Geometry check sheet. Reference: drawing and pictorial views, mm from the part's lowest x, y, z. A direction names the side the tool comes from. Give positions to 0.01 mm unless a question says otherwise; leave off trailing zeros. Write each loop counter-clockwise with the first axis right and the second up, starting at its lowest first coordinate (ties: lowest second). Pieces come first, ordered by that corner, then holes.
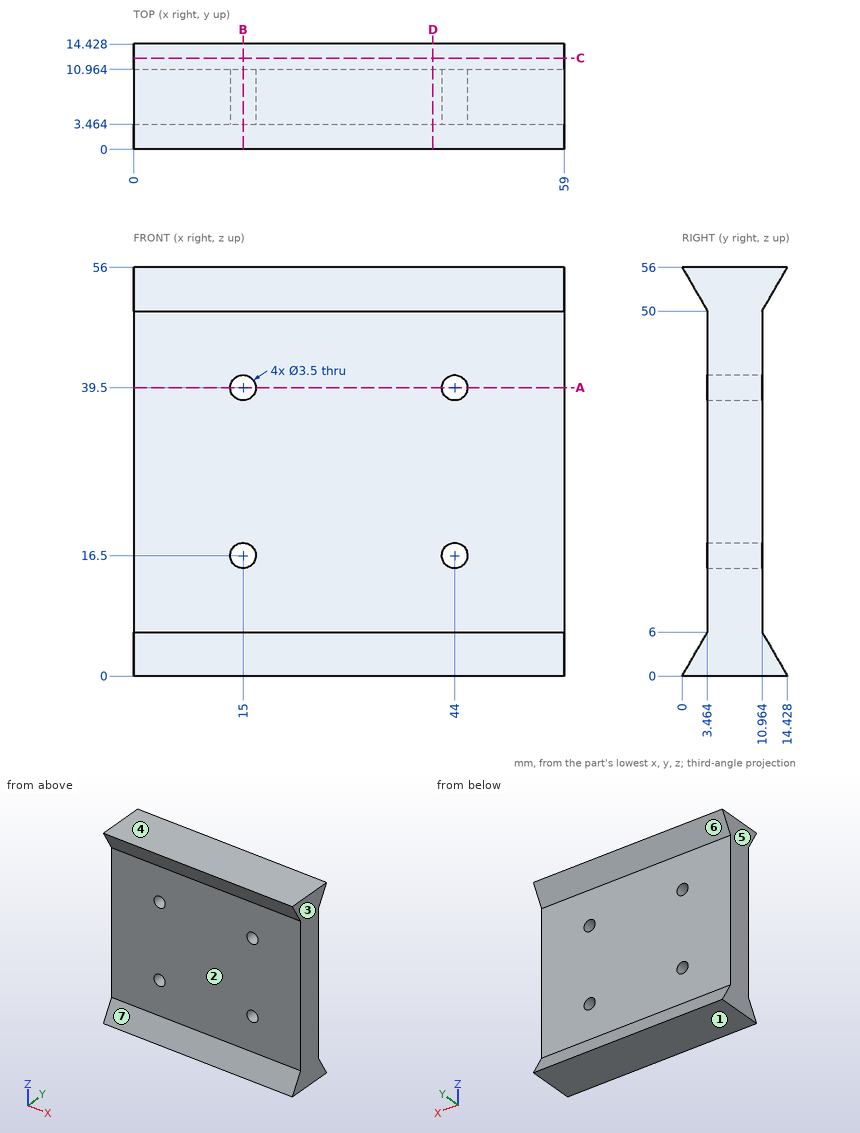
Item 1: Sectioned sample at D-D on x = 41. Record the cut outline in (y, z).
Answer key:
outline: (0, 0) - (14.43, 0) - (10.96, 6) - (10.96, 50) - (14.43, 56) - (0, 56) - (3.46, 50) - (3.46, 6) - close
Item 2: Depth check by flat-ended pin: pin 1 (4.5 mm diameter, centred on x = 15, z = 39.5, fed in from +Y); pin 2 (5 mm diameter, centred on x = 27, z = 26.5, fed in from -Y). Enter the tip coordinate at first touch or a pass-through.
Answer key:
pin 1: stops at y = 10.96
pin 2: stops at y = 3.46
Item 3: Sectioned sample at B-B on x = 15. Record the cut outline in (y, z).
Answer key:
outline: (0, 0) - (14.43, 0) - (10.96, 6) - (10.96, 14.75) - (3.46, 14.75) - (3.46, 6) - close; (0, 56) - (3.46, 50) - (3.46, 41.25) - (10.96, 41.25) - (10.96, 50) - (14.43, 56) - close; (3.46, 18.25) - (10.96, 18.25) - (10.96, 37.75) - (3.46, 37.75) - close
Item 4: Sectioned sample at A-A on z = 39.5. Record the cut outline in (x, y).
Answer key:
outline: (0, 3.46) - (13.25, 3.46) - (13.25, 10.96) - (0, 10.96) - close; (16.75, 3.46) - (42.25, 3.46) - (42.25, 10.96) - (16.75, 10.96) - close; (45.75, 3.46) - (59, 3.46) - (59, 10.96) - (45.75, 10.96) - close
Item 5: Scan lines: line 1 along X through (y, z) = (5.5, 16.5); line 2 along X through (y, z) = (9.75, 38); line 3 along Y through (x, z) = (33, 36.5). Record each from-to range of solid material in increasing order.
Answer key:
line 1: x = 0 to 13.25, 16.75 to 42.25, 45.75 to 59
line 2: x = 0 to 14.1, 15.9 to 43.1, 44.9 to 59
line 3: y = 3.46 to 10.96
Item 6: Sectioned sample at C-C on y = 12.5. Record the cut outline in (x, z).
Answer key:
outline: (0, 0) - (59, 0) - (59, 3.34) - (0, 3.34) - close; (0, 52.66) - (59, 52.66) - (59, 56) - (0, 56) - close
Item 7: Set-up check for the marked faces 5, 6 and 7: record each of +Z, -Z, +X, -X, +Y, -Y from which the full face is reachable in a straight line by a thin tool's end or side.
Answer key:
face 5: +Z, -Z, -X, +Y, -Y
face 6: +X, -X, +Y
face 7: +X, -X, -Y
Item 8: Release check for a two-part mould opening along Z. For the marked faces 1, 2, 3 and 4 record: released by +Z, released by -Z, zero draft, split by the parting line, or undercut.
Answer key:
face 1: released by -Z
face 2: undercut
face 3: zero draft
face 4: released by +Z
